Model file for the job. Use its own axes, mm. A direction names the side the tool comes from. Round coordinates to 2 decimals unless told otherwise and drop trailing zeros. Loops run counter-clockwise (first coordinate to the right, second up) from the corner with the lowest first, then second, coordinate; pieces in that order, holes last. Notation, with made-up numbers: (-32.75, -18) - (-16.75, -18) arc R18 ccw to (-16.75, -10) - close; hole circle Ø1 at (41, 16.5). An arc over 180 degrees is marked (long way). Answer as a JSON object with one key per item and string values.
from build123d import *

# Parameters (mm, degrees)
F0_R     = 10
F0_R_2   = 3
F0_R_3   = 5
F0_R_4   = 4
F1_DEPTH = 10
F2_R     = 1
F3_DEPTH = 9


with BuildPart() as f1:
    # F0 (on Front) → F1 (new body)
    with BuildSketch(Plane.XZ):
        with BuildLine():
            Line((195.5, -25), (204.1, -25))
            ThreePointArc((204.1, -25), (225.169837, -8.939366), (251, -3.05))
            Line((251, -3.05), (251, 3.05))
            ThreePointArc((251, 3.05), (225.169837, 8.939366), (204.1, 25))
            Line((204.1, 25), (195.5, 25))
            Line((195.5, 25), (195.5, 21))
            Line((195.5, 21), (-195.5, 21))
            Line((-195.5, 21), (-195.5, 25))
            Line((-195.5, 25), (-204.1, 25))
            ThreePointArc((-204.1, 25), (-225.169837, 8.939366), (-251, 3.05))
            Line((-251, 3.05), (-251, -3.05))
            ThreePointArc((-251, -3.05), (-225.169837, -8.939366), (-204.1, -25))
            Line((-204.1, -25), (-195.5, -25))
            Line((-195.5, -25), (-195.5, -21))
            Line((-195.5, -21), (195.5, -21))
            Line((195.5, -21), (195.5, -25))
        make_face()
        with BuildLine():
            Line((-202.64971, 21.81), (-198.69, 21.81))
            Line((-198.69, 21.81), (-198.69, 17.81))
            Line((-198.69, 17.81), (198.69, 17.81))
            Line((198.69, 17.81), (198.69, 21.81))
            Line((198.69, 21.81), (202.64971, 21.81))
            ThreePointArc((202.64971, 21.81), (222.843542, 6.515825), (247.323057, 0))
            ThreePointArc((247.323057, 0), (222.843542, -6.515825), (202.64971, -21.81))
            Line((202.64971, -21.81), (198.69, -21.81))
            Line((198.69, -21.81), (198.69, -17.81))
            Line((198.69, -17.81), (-198.69, -17.81))
            Line((-198.69, -17.81), (-198.69, -21.81))
            Line((-198.69, -21.81), (-202.64971, -21.81))
            ThreePointArc((-202.64971, -21.81), (-222.843542, -6.515825), (-247.323057, 0))
            ThreePointArc((-247.323057, 0), (-222.843542, 6.515825), (-202.64971, 21.81))
        make_face(mode=Mode.SUBTRACT)
        with BuildLine():
            Line((202.203828, 20.81), (199.69, 20.81))
            Line((199.69, 20.81), (199.69, 16.81))
            Line((199.69, 16.81), (-199.69, 16.81))
            Line((-199.69, 16.81), (-199.69, 20.81))
            Line((-199.69, 20.81), (-202.203828, 20.81))
            ThreePointArc((-202.203828, 20.81), (-219.078949, 7.358512), (-239.366002, 0))
            ThreePointArc((-239.366002, 0), (-219.078949, -7.358512), (-202.203828, -20.81))
            Line((-202.203828, -20.81), (-199.69, -20.81))
            Line((-199.69, -20.81), (-199.69, -16.81))
            Line((-199.69, -16.81), (199.69, -16.81))
            Line((199.69, -16.81), (199.69, -20.81))
            Line((199.69, -20.81), (202.203828, -20.81))
            ThreePointArc((202.203828, -20.81), (219.078949, -7.358512), (239.366002, 0))
            ThreePointArc((239.366002, 0), (219.078949, 7.358512), (202.203828, 20.81))
        make_face()
        with Locations((-201, 0)):
            Circle(F0_R, mode=Mode.SUBTRACT)
        with Locations((-152, 0)):
            Circle(F0_R_2, mode=Mode.SUBTRACT)
        with Locations((-109.6, 0)):
            Circle(F0_R_3, mode=Mode.SUBTRACT)
        with Locations((-71, 0)):
            Circle(F0_R_2, mode=Mode.SUBTRACT)
        with Locations((-34.8, 0)):
            Circle(F0_R_4, mode=Mode.SUBTRACT)
        with Locations((16.5, 0)):
            Circle(F0_R_2, mode=Mode.SUBTRACT)
        with Locations((62.5, 0)):
            Circle(F0_R_2, mode=Mode.SUBTRACT)
        with Locations((103.2, 0)):
            Circle(F0_R_2, mode=Mode.SUBTRACT)
        with Locations((142.5, 0)):
            Circle(F0_R_3, mode=Mode.SUBTRACT)
        with Locations((194.1, 0)):
            Circle(F0_R, mode=Mode.SUBTRACT)
    extrude(amount=F1_DEPTH)

    # F2
    f2_edges = [f1.edges().sort_by_distance(p)[0] for p in [
        (0, -10, 21),
        (-195.5, -10, 23),
        (-251, -10, 0),
        (-225.169837, -10, -8.939366),
        (-199.8, -10, -25),
        (-195.5, -10, -23),
        (0, -10, -21),
        (195.5, -10, -23),
        (199.8, -10, -25),
        (225.169837, -10, -8.939366),
        (251, -10, 0),
        (225.169837, -10, 8.939366),
        (199.8, -10, 25),
        (195.5, -10, 23),
        (-199.8, -10, 25),
        (-225.169837, -10, 8.939366),
    ]]
    fillet(f2_edges, radius=F2_R)

    # F0 (on Front) → F3 (join)
    with BuildSketch(Plane.XZ):
        with BuildLine():
            Line((-198.69, 17.81), (-198.69, 21.81))
            Line((-198.69, 21.81), (-202.64971, 21.81))
            ThreePointArc((-202.64971, 21.81), (-222.843542, 6.515825), (-247.323057, 0))
            ThreePointArc((-247.323057, 0), (-222.843542, -6.515825), (-202.64971, -21.81))
            Line((-202.64971, -21.81), (-198.69, -21.81))
            Line((-198.69, -21.81), (-198.69, -17.81))
            Line((-198.69, -17.81), (198.69, -17.81))
            Line((198.69, -17.81), (198.69, -21.81))
            Line((198.69, -21.81), (202.64971, -21.81))
            ThreePointArc((202.64971, -21.81), (222.843542, -6.515825), (247.323057, 0))
            ThreePointArc((247.323057, 0), (222.843542, 6.515825), (202.64971, 21.81))
            Line((202.64971, 21.81), (198.69, 21.81))
            Line((198.69, 21.81), (198.69, 17.81))
            Line((198.69, 17.81), (-198.69, 17.81))
        make_face()
        with BuildLine():
            Line((199.69, 16.81), (199.69, 20.81))
            Line((199.69, 20.81), (202.203828, 20.81))
            ThreePointArc((202.203828, 20.81), (219.078949, 7.358512), (239.366002, 0))
            ThreePointArc((239.366002, 0), (219.078949, -7.358512), (202.203828, -20.81))
            Line((202.203828, -20.81), (199.69, -20.81))
            Line((199.69, -20.81), (199.69, -16.81))
            Line((199.69, -16.81), (-199.69, -16.81))
            Line((-199.69, -16.81), (-199.69, -20.81))
            Line((-199.69, -20.81), (-202.203828, -20.81))
            ThreePointArc((-202.203828, -20.81), (-219.078949, -7.358512), (-239.366002, 0))
            ThreePointArc((-239.366002, 0), (-219.078949, 7.358512), (-202.203828, 20.81))
            Line((-202.203828, 20.81), (-199.69, 20.81))
            Line((-199.69, 20.81), (-199.69, 16.81))
            Line((-199.69, 16.81), (199.69, 16.81))
        make_face(mode=Mode.SUBTRACT)
    extrude(amount=F3_DEPTH)


solid = f1.part
1) Probe probe 1 along Z at (x, y) = (-152, -5.5); probe 2 along Z at (x, y) = (-34.8, -6.5); probe 3 along Z at (x, y) = (220, -9.5). List the from-to ranges inside material, lowest first.
Values follow:
{"probe 1": "-21 to -3, 3 to 21", "probe 2": "-21 to -4, 4 to 21", "probe 3": "-11.51 to -7.99, -6.85 to 6.85, 7.99 to 11.51"}
2) Drop flat-ended pins along their axis: P1, Ø1.1, axis at y = -9.5, z = 19.5, coming from the -X side; P2, Ø4, axis at x = -98.5, y = -6.5, coming from the +Z side; P3, Ø1.1, axis at x = 67, y = -9.5, coming from the -Z side. Give the stop position or say it passes through.
Values follow:
{"P1": "x = -209.9", "P2": "z = 21", "P3": "z = -21"}
3) Two-plate mould, pull along Z, no slides. Class faces 1 (the flat face through (200, -4, 25)), 2 (the cylindrical face through (-218.81, -9.49, 7.51)), 3 (the flat face through (200, -4, -25)), 4 (the cylindrical face through (218.81, -9.49, -7.51)): pulls with the +Z half, pulls with the -Z half, needs draft (parallel to the pull), parting line crosses it, or undercut.
Values follow:
{"face 1": "pulls with the +Z half", "face 2": "undercut", "face 3": "pulls with the -Z half", "face 4": "undercut"}
4) Slice it at C-C on x = -109.6. List the corners of the cut face in (y, z).
Values follow:
{"outline": "(-10, -20) arc R1 ccw to (-9, -21) - (0, -21) - (0, -5) - (-10, -5) - (-10, -16.81) - (-9, -16.81) - (-9, -17.81) - (-10, -17.81) - close; (-10, 5) - (0, 5) - (0, 21) - (-9, 21) arc R1 ccw to (-10, 20) - (-10, 17.81) - (-9, 17.81) - (-9, 16.81) - (-10, 16.81) - close"}
5) Slice it at B-B on y = -2. Count the separate pieces of the cut face and the enclosed holes in it, then the cut area to 3 significant figures.
Values follow:
{"separate pieces": "1", "enclosed holes": "10", "area": "18,200 mm²"}
6) Slice it at A-A on x = -1. List the corners of the cut face in (y, z).
Values follow:
{"outline": "(-10, -20) arc R1 ccw to (-9, -21) - (0, -21) - (0, 21) - (-9, 21) arc R1 ccw to (-10, 20) - (-10, 17.81) - (-9, 17.81) - (-9, 16.81) - (-10, 16.81) - (-10, -16.81) - (-9, -16.81) - (-9, -17.81) - (-10, -17.81) - close"}
7) Tool access for faces 5 (the cylindrical face through (-219.344, -9.493, -7.211)), 6 (the flat face through (-200, -4, 25)), 7 (the flat face through (3, -4, 21)): list every direction of +Z, -Z, +X, -X, +Y, -Y with a clear straight run to the whole face (end or side of a thin tool).
Values follow:
{"face 5": "-Y", "face 6": "+Z, +X, -X, +Y, -Y", "face 7": "+Z, +Y, -Y"}
